Check sheet for the drawn part. Datum: minimum x, y, z corner. Units: mm. A direction names the side the tool comes from. Give positions to 0.01 mm unless a question says otherwise; leave off trailing zeros. Order: outer loops, then holes, each group sorted by start corner. A loop starts at its lowest first (then second) coordinate and runs counter-clockwise, first axis right, second up. Notation, with made-up numbers: M -11,14.25 L 29,14.25 A27 cw 29,37.25 Z; hole C 43,-31.5 d10. An arc over 180 degrees is marked long. Answer in a Markdown table with one row per item. Add a question column.
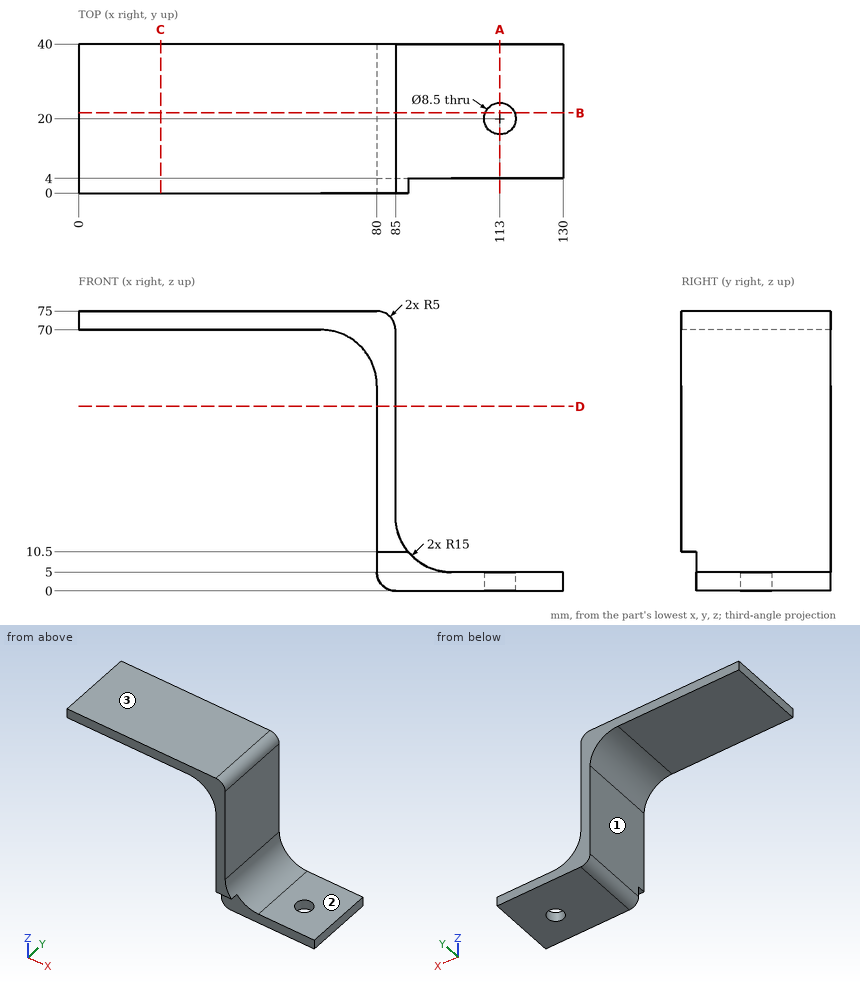
Q1. Tool access check on the marked faces 1, 2 and 3. Record the directions out of +Z, -Z, +X, -X, +Y, -Y that give a thin tool (end or side, any length) a straight path to the whole face; none if there is none.
Q2. Thickness scan on probe 1 along Y at (x, z) = (113, 2.8); probe 2 along Z at (x, y) = (19.5, 8); probe 3 along X at (y, z) = (32.5, 32). Record the ranges inside material, lowest first.
Q3. Cross-section at D-D (z = 49.5). Record the boundary of the cut face in (x, y).
Q4. Cross-section at C-C (x = 22). Record the boundary of the cut face in (y, z), and give its area (3 significant figures).
Q5. Go/stop test with flat-tipped pins: pin 1 (1.5 mm diameter, centred on y = 14, z = 35.5, fed in from +X); pin 2 (1 mm diameter, centred on y = 7, z = 52, fed in from -X); pin 3 (8.5 mm diameter, centred on x = 97, z = 7, fed in from -Y); pin 4 (10 mm diameter, centred on x = 91.5, z = 17, fed in from +Y). Record where each tip stops, or that it passes through.
Q6. Cross-section at A-A (x = 113). Record the boundary of the cut face in (y, z).
Q7. Cross-section at B-B (y = 21.5). Record the boundary of the cut face in (x, z).
Values follow:
| question | item | result |
|---|---|---|
| 1 | face 1 | -Z, -X, +Y, -Y |
| 1 | face 2 | +Z, +X, +Y, -Y |
| 1 | face 3 | +Z, +X, -X, +Y, -Y |
| 2 | probe 1 | 4 to 15.75, 24.25 to 40 |
| 2 | probe 2 | 70 to 75 |
| 2 | probe 3 | 80 to 85 |
| 3 | outline | M 80,0 L 85,0 L 85,40 L 80,40 Z |
| 4 | outline | M 0,70 L 40,70 L 40,75 L 0,75 Z |
| 4 | area | 200 mm² |
| 5 | pin 1 | x = 85 |
| 5 | pin 2 | x = 80 |
| 5 | pin 3 | y = 4 |
| 5 | pin 4 | through |
| 6 | outline | M 4,0 L 15.75,0 L 15.75,5 L 4,5 Z; M 24.25,0 L 40,0 L 40,5 L 24.25,5 Z |
| 7 | outline | M 0,70 L 65,70 A15 cw 80,55 L 80,5 A5 ccw 85,0 L 109.02,0 L 109.02,5 L 100,5 A15 cw 85,20 L 85,70 A5 ccw 80,75 L 0,75 Z; M 116.98,0 L 130,0 L 130,5 L 116.98,5 Z |
